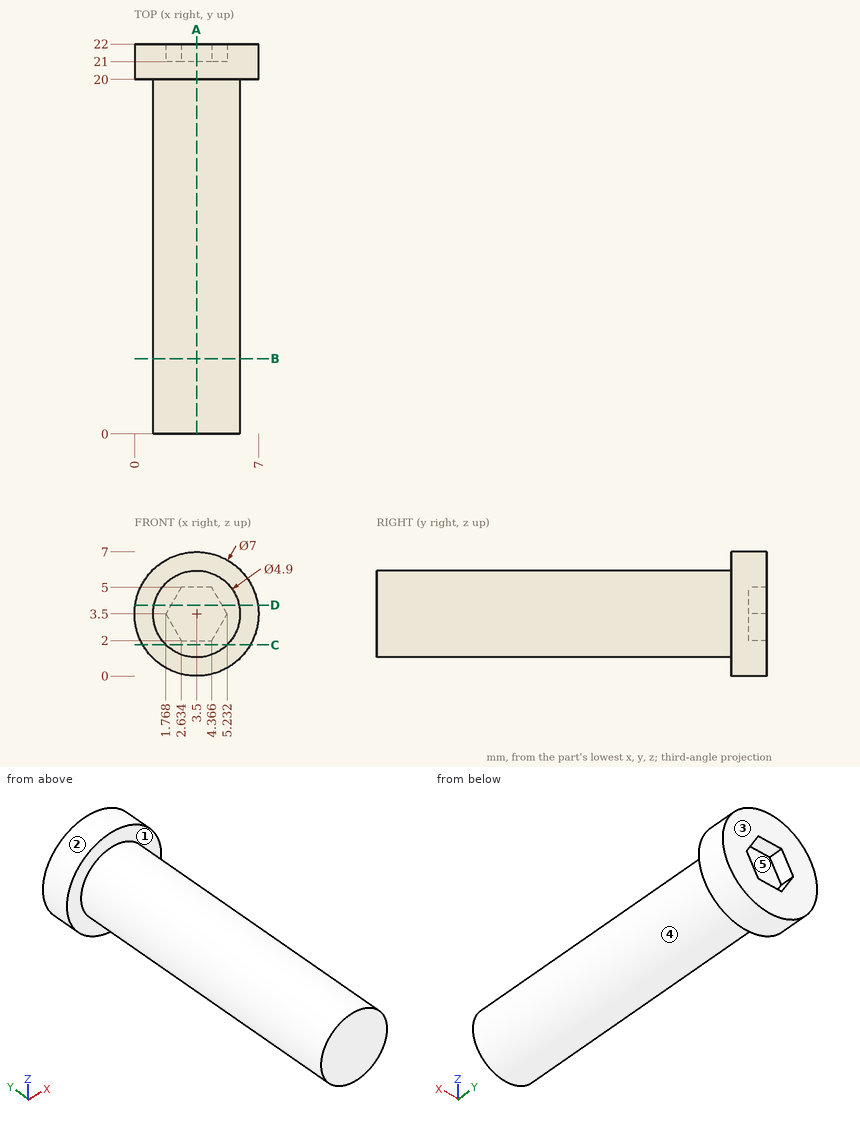
Geometry: see drawing. Coordinates: mm, zero at the bounding-box minimum. A direction names the side the tool comes from. Give positions to 0.01 mm unless a question says otherwise; leave off trailing zeros. Order: outer loops, then holes, each group sorted by start corner. A loop starts at its lowest first (then second) coordinate and runs counter-clockwise, first axis right, second up. Notation, with made-up numbers: (2.25, -19) - (28.25, -19) arc R20 cw to (28.25, -3) - close; hole circle Ø3 at (52, 5). An arc over 180 degrees is marked (long way). Use CSV: the item, a comma, the result in double quotes.
1. Section query A-A (x = 3.5). Output: boundary loops of the cut face in (y, z), plus the area to 3 significant figures.
Answers below:
outline,"(0, 1.05) - (20, 1.05) - (20, 0) - (22, 0) - (22, 2) - (21, 2) - (21, 5) - (22, 5) - (22, 7) - (20, 7) - (20, 5.95) - (0, 5.95) - close"
area,"109 mm2"
2. Contact query for flat-ended pins moving along their axis: pin 1 (1 mm diameter, centred on y = 16.5, z = 2.5, fed in from +X); pin 2 (2.5 mm diameter, centred on x = 3.5, z = 3, fed in from +Y); pin 3 (1.5 mm diameter, centred on x = 5.5, y = 8, fed in from -Z). Output: stop coordinate, or through.
Answers below:
pin 1,"x = 5.9"
pin 2,"y = 22"
pin 3,"z = 1.39"
3. Material intervals for line 1 along Y through (x, z) = (1.5, 1.25); line 2 along Y through (x, z) = (3.5, 4); line 3 along X through (y, z) = (17, 3), sorted ascending. Write a range as from..to.
Answers below:
line 1,"20..22"
line 2,"0..21"
line 3,"1.1..5.9"
4. Section query B-B (y = 4.25). Output: boundary loops of the cut face in (x, z).
Answers below:
outline,"circle Ø4.9 at (3.5, 3.5)"
5. Access query for the marked faces 1 and 2. Directions: +Z, -Z, +X, -X, +Y, -Y. A direction counts if a zero-diameter tool reaches every point of the face in a straight line with its end or side. Return the directions, or none.
Answers below:
face 1,"-Y"
face 2,"+Y, -Y"
6. Mould query, pull axis Z, two halves, no side actions, for the marked faces 3, 4 and 5. Classes: +Z half, -Z half, draft (parallel to the pull), parting line (faces both ways), or undercut.
Answers below:
face 3,"draft"
face 4,"parting line"
face 5,"undercut"
7. Section query D-D (z = 4). Output: boundary loops of the cut face in (x, y).
Answers below:
outline,"(0.04, 20) - (1.1, 20) - (1.1, 0) - (5.9, 0) - (5.9, 20) - (6.96, 20) - (6.96, 22) - (4.94, 22) - (4.94, 21) - (2.06, 21) - (2.06, 22) - (0.04, 22) - close"
8. Section query C-C (z = 1.75). Output: boundary loops of the cut face in (x, y), plus the area to 3 significant figures.
Answers below:
outline,"(0.47, 20) - (1.79, 20) - (1.79, 0) - (5.21, 0) - (5.21, 20) - (6.53, 20) - (6.53, 22) - (0.47, 22) - close"
area,"80.7 mm2"
